Check sheet for the modelled part. Datum: model origin and axes. Units: mm. Face numbers are marked on the shaded views. A direction names the side the tool comes from. Coordinates: 2 decimals unless noted, no trailing zeros. Loops run counter-clockwise (first coordinate to the right, second up) from the corner with the lowest first, then second, coordinate; pieces in that order, holes last. Notation, with made-up numbers: (85.25, 49) -> (112.25, 49) arc R29 cw to (112.25, 77) -> close; hole circle Ø6 at (8.25, 2.25). An arc over 180 degrees is marked (long way). Use one line per item in the form item = value.
from build123d import *

# Parameters (mm, degrees)
SKETCH1_R           = 10
BOSS_EXTRUDE1_DEPTH = 10
BOSS_EXTRUDE2_DEPTH = 10
SKETCH4_R           = 2.825
CUT_EXTRUDE1_DEPTH  = 3.7
SKETCH5_R           = 1.6
CUT_EXTRUDE2_DEPTH  = 20.917820636
SKETCH7_R           = 3
CUT_EXTRUDE3_DEPTH  = 3


with BuildPart() as part:
    # Sketch1 → Boss-Extrude1 (new body)
    with BuildSketch(Plane(origin=(0, 0, 0), x_dir=(1, 0, 0), z_dir=(0, 1, 0))):
        with Locations(Location((0, 0, 0), (0, 0, 270))):
            Circle(SKETCH1_R)
    extrude(amount=BOSS_EXTRUDE1_DEPTH)

    # Sketch3 → Boss-Extrude2 (add)
    with BuildSketch(Plane(origin=(0, 10, 0), x_dir=(1, 0, 0), z_dir=(0, 1, 0))):
        with BuildLine():
            ThreePointArc((-0.292653692, 12.182759316), (-0.746983902, 11.075453202), (-0.972488982, 9.9))
            ThreePointArc((-0.972488982, 9.9), (0, 9.947649713), (0.972488982, 9.9))
            ThreePointArc((0.972488982, 9.9), (0.746983902, 11.075453202), (0.292653692, 12.182759316))
            ThreePointArc((0.292653692, 12.182759316), (0, 12.186273866), (-0.292653692, 12.182759316))
        make_face()
        with BuildLine():
            ThreePointArc((3.005067828, 11.809946574), (2.2688378, 10.866279198), (1.734561582, 9.795255532))
            ThreePointArc((1.734561582, 9.795255532), (2.683843773, 9.578763877), (3.607414487, 9.270506757))
            ThreePointArc((3.607414487, 9.270506757), (3.707405226, 10.463211508), (3.568670426, 11.652032532))
            ThreePointArc((3.568670426, 11.652032532), (3.287817341, 11.734373774), (3.005067828, 11.809946574))
        make_face()
        with BuildLine():
            ThreePointArc((6.079917215, 10.561244121), (5.116390182, 9.851202976), (4.312967649, 8.964041772))
            ThreePointArc((4.312967649, 8.964041772), (5.168639132, 8.499464945), (5.974794562, 7.953462438))
            ThreePointArc((5.974794562, 7.953462438), (6.392865264, 9.074961283), (6.580015201, 10.257127799))
            ThreePointArc((6.580015201, 10.257127799), (6.331792311, 10.41218886), (6.079917215, 10.561244121))
        make_face()
        with BuildLine():
            ThreePointArc((8.703846955, 8.529262507), (7.58448331, 8.105508096), (6.571500635, 7.468006041))
            ThreePointArc((6.571500635, 7.468006041), (7.270100171, 6.789799579), (7.899051458, 6.046546195))
            ThreePointArc((7.899051458, 6.046546195), (8.604195731, 7.013662695), (9.103350349, 8.101498821))
            ThreePointArc((9.103350349, 8.101498821), (8.906167212, 8.317779531), (8.703846955, 8.529262507))
        make_face()
        with BuildLine():
            ThreePointArc((10.682252184, 5.864704511), (9.490070008, 5.758664761), (8.342655482, 5.418102466))
            ThreePointArc((8.342655482, 5.418102466), (8.832371138, 4.576565841), (9.237471842, 3.691185281))
            ThreePointArc((9.237471842, 3.691185281), (10.177392362, 4.43219283), (10.951531647, 5.345018737))
            ThreePointArc((10.951531647, 5.345018737), (10.820012433, 5.606478546), (10.682252184, 5.864704511))
        make_face()
        with BuildLine():
            ThreePointArc((11.868403637, 2.765188211), (10.691821627, 2.984727604), (9.495073737, 2.966363017))
            ThreePointArc((9.495073737, 2.966363017), (9.739585544, 2.02390915), (9.890791199, 1.062066042))
            ThreePointArc((9.890791199, 1.062066042), (10.99577836, 1.522007499), (11.987487943, 2.192123066))
            ThreePointArc((11.987487943, 2.192123066), (11.93138683, 2.479370695), (11.868403637, 2.765188211))
        make_face()
        with BuildLine():
            ThreePointArc((12.174329886, -0.539409449), (11.100609748, -0.010573145), (9.94328581, 0.294621993))
            ThreePointArc((9.94328581, 0.294621993), (9.924459446, -0.678851624), (9.81055582, -1.645821778))
            ThreePointArc((9.81055582, -1.645821778), (10.99865778, -1.501058166), (12.134387098, -1.123352345))
            ThreePointArc((12.134387098, -1.123352345), (12.157864849, -0.831620739), (12.174329886, -0.539409449))
        make_face()
        with BuildLine():
            ThreePointArc((11.577341782, -3.804001578), (10.686116426, -3.005089732), (9.654049862, -2.398969796))
            ThreePointArc((9.654049862, -2.398969796), (9.373281592, -3.331265078), (9.002716396, -4.231646525))
            ThreePointArc((9.002716396, -4.231646525), (10.185817067, -4.412797214), (11.381334272, -4.355513852))
            ThreePointArc((11.381334272, -4.355513852), (11.48264965, -4.080934666), (11.577341782, -3.804001578))
        make_face()
        with BuildLine():
            ThreePointArc((10.1217152, -6.786468311), (9.479082735, -5.776732561), (8.6488172, -4.914640969))
            ThreePointArc((8.6488172, -4.914640969), (8.126930322, -5.736613841), (7.527186681, -6.503629408))
            ThreePointArc((7.527186681, -6.503629408), (8.6175409, -6.997259279), (9.78417995, -7.264646822))
            ThreePointArc((9.78417995, -7.264646822), (9.955818856, -7.027584338), (10.1217152, -6.786468311))
        make_face()
        with BuildLine():
            ThreePointArc((7.915407306, -9.265613737), (7.569028841, -8.119941563), (7.002141332, -7.065815706))
            ThreePointArc((7.002141332, -7.065815706), (6.277841808, -7.716504199), (5.493399966, -8.29326785))
            ThreePointArc((5.493399966, -8.29326785), (6.410141146, -9.062766634), (7.46137776, -9.63499417))
            ThreePointArc((7.46137776, -9.63499417), (7.690610523, -9.453030229), (7.915407306, -9.265613737))
        make_face()
        with BuildLine():
            ThreePointArc((5.122049862, -11.057570978), (5.097614704, -9.860931645), (4.836148674, -8.692951215))
            ThreePointArc((4.836148674, -8.692951215), (3.963154487, -9.124096741), (3.052192905, -9.467832555))
            ThreePointArc((3.052192905, -9.467832555), (3.727330549, -10.456130047), (4.585199315, -11.290758078))
            ThreePointArc((4.585199315, -11.290758078), (4.855024789, -11.177388113), (5.122049862, -11.057570978))
        make_face()
        with BuildLine():
            ThreePointArc((1.948813412, -12.029438766), (2.248133804, -10.870581538), (2.311480993, -9.6753703))
            ThreePointArc((2.311480993, -9.6753703), (1.354538128, -9.854996767), (0.384618659, -9.940211432))
            ThreePointArc((0.384618659, -9.940211432), (0.768080896, -11.074010128), (1.368957613, -12.109138111))
            ThreePointArc((1.368957613, -12.109138111), (1.659364077, -12.072770253), (1.948813412, -12.029438766))
        make_face()
        with BuildLine():
            ThreePointArc((-1.368957613, -12.109138111), (-0.768080896, -11.074010128), (-0.384618659, -9.940211432))
            ThreePointArc((-0.384618659, -9.940211432), (-1.354538128, -9.854996767), (-2.311480993, -9.6753703))
            ThreePointArc((-2.311480993, -9.6753703), (-2.248133804, -10.870581538), (-1.948813412, -12.029438766))
            ThreePointArc((-1.948813412, -12.029438766), (-1.659364077, -12.072770253), (-1.368957613, -12.109138111))
        make_face()
        with BuildLine():
            ThreePointArc((-4.585199315, -11.290758078), (-3.727330549, -10.456130047), (-3.052192905, -9.467832555))
            ThreePointArc((-3.052192905, -9.467832555), (-3.963154487, -9.124096741), (-4.836148674, -8.692951215))
            ThreePointArc((-4.836148674, -8.692951215), (-5.097614704, -9.860931645), (-5.122049862, -11.057570978))
            ThreePointArc((-5.122049862, -11.057570978), (-4.855024789, -11.177388113), (-4.585199315, -11.290758078))
        make_face()
        with BuildLine():
            ThreePointArc((-7.46137776, -9.63499417), (-6.410141146, -9.062766634), (-5.493399966, -8.29326785))
            ThreePointArc((-5.493399966, -8.29326785), (-6.277841808, -7.716504199), (-7.002141332, -7.065815706))
            ThreePointArc((-7.002141332, -7.065815706), (-7.569028841, -8.119941563), (-7.915407306, -9.265613737))
            ThreePointArc((-7.915407306, -9.265613737), (-7.690610523, -9.453030229), (-7.46137776, -9.63499417))
        make_face()
        with BuildLine():
            ThreePointArc((-9.78417995, -7.264646822), (-8.6175409, -6.997259279), (-7.527186681, -6.503629408))
            ThreePointArc((-7.527186681, -6.503629408), (-8.126930322, -5.736613841), (-8.6488172, -4.914640969))
            ThreePointArc((-8.6488172, -4.914640969), (-9.479082735, -5.776732561), (-10.1217152, -6.786468311))
            ThreePointArc((-10.1217152, -6.786468311), (-9.955818856, -7.027584338), (-9.78417995, -7.264646822))
        make_face()
        with BuildLine():
            ThreePointArc((-11.381334272, -4.355513852), (-10.185817067, -4.412797214), (-9.002716396, -4.231646525))
            ThreePointArc((-9.002716396, -4.231646525), (-9.373281592, -3.331265078), (-9.654049862, -2.398969796))
            ThreePointArc((-9.654049862, -2.398969796), (-10.686116426, -3.005089732), (-11.577341782, -3.804001578))
            ThreePointArc((-11.577341782, -3.804001578), (-11.48264965, -4.080934666), (-11.381334272, -4.355513852))
        make_face()
        with BuildLine():
            ThreePointArc((-12.134387098, -1.123352345), (-10.99865778, -1.501058166), (-9.81055582, -1.645821778))
            ThreePointArc((-9.81055582, -1.645821778), (-9.924459446, -0.678851624), (-9.94328581, 0.294621993))
            ThreePointArc((-9.94328581, 0.294621993), (-11.100609748, -0.010573145), (-12.174329886, -0.539409449))
            ThreePointArc((-12.174329886, -0.539409449), (-12.157864849, -0.831620739), (-12.134387098, -1.123352345))
        make_face()
        with BuildLine():
            ThreePointArc((-11.987487943, 2.192123066), (-10.99577836, 1.522007499), (-9.890791199, 1.062066042))
            ThreePointArc((-9.890791199, 1.062066042), (-9.739585544, 2.02390915), (-9.495073737, 2.966363017))
            ThreePointArc((-9.495073737, 2.966363017), (-10.691821627, 2.984727604), (-11.868403637, 2.765188211))
            ThreePointArc((-11.868403637, 2.765188211), (-11.93138683, 2.479370695), (-11.987487943, 2.192123066))
        make_face()
        with BuildLine():
            ThreePointArc((-10.951531647, 5.345018737), (-10.177392362, 4.43219283), (-9.237471842, 3.691185281))
            ThreePointArc((-9.237471842, 3.691185281), (-8.832371138, 4.576565841), (-8.342655482, 5.418102466))
            ThreePointArc((-8.342655482, 5.418102466), (-9.490070008, 5.758664761), (-10.682252184, 5.864704511))
            ThreePointArc((-10.682252184, 5.864704511), (-10.820012433, 5.606478546), (-10.951531647, 5.345018737))
        make_face()
        with BuildLine():
            ThreePointArc((-9.103350349, 8.101498821), (-8.604195731, 7.013662695), (-7.899051458, 6.046546195))
            ThreePointArc((-7.899051458, 6.046546195), (-7.270100171, 6.789799579), (-6.571500635, 7.468006041))
            ThreePointArc((-6.571500635, 7.468006041), (-7.58448331, 8.105508096), (-8.703846955, 8.529262507))
            ThreePointArc((-8.703846955, 8.529262507), (-8.906167212, 8.317779531), (-9.103350349, 8.101498821))
        make_face()
        with BuildLine():
            ThreePointArc((-6.580015201, 10.257127799), (-6.392865264, 9.074961283), (-5.974794562, 7.953462438))
            ThreePointArc((-5.974794562, 7.953462438), (-5.168639132, 8.499464945), (-4.312967649, 8.964041772))
            ThreePointArc((-4.312967649, 8.964041772), (-5.116390182, 9.851202976), (-6.079917215, 10.561244121))
            ThreePointArc((-6.079917215, 10.561244121), (-6.331792311, 10.41218886), (-6.580015201, 10.257127799))
        make_face()
        with BuildLine():
            ThreePointArc((-3.568670426, 11.652032532), (-3.707405226, 10.463211508), (-3.607414487, 9.270506757))
            ThreePointArc((-3.607414487, 9.270506757), (-2.683843773, 9.578763877), (-1.734561582, 9.795255532))
            ThreePointArc((-1.734561582, 9.795255532), (-2.2688378, 10.866279198), (-3.005067828, 11.809946574))
            ThreePointArc((-3.005067828, 11.809946574), (-3.287817341, 11.734373774), (-3.568670426, 11.652032532))
        make_face()
    extrude(amount=-BOSS_EXTRUDE2_DEPTH)

    # Sketch4 → Cut-Extrude1 (cut)
    with BuildSketch(Plane.XZ):
        with Locations(Location((0, 0, 0), (0, 0, 270))):
            Circle(SKETCH4_R)
    extrude(amount=-CUT_EXTRUDE1_DEPTH, mode=Mode.SUBTRACT)

    # Sketch5 → Cut-Extrude2 (cut, through all)
    with BuildSketch(Plane(origin=(0, 10, 0), x_dir=(1, 0, 0), z_dir=(0, 1, 0))):
        with Locations(Location((0, 0, 0), (0, 0, 270))):
            Circle(SKETCH5_R)
    extrude(amount=-CUT_EXTRUDE2_DEPTH, mode=Mode.SUBTRACT)

    # Sketch7 → Cut-Extrude3 (cut)
    with BuildSketch(Plane(origin=(0, 10, 0), x_dir=(1, 0, 0), z_dir=(0, 1, 0))):
        with Locations(Location((0, 0, 0), (0, 0, 270))):
            Circle(SKETCH7_R)
    extrude(amount=-CUT_EXTRUDE3_DEPTH, mode=Mode.SUBTRACT)


solid = part.part
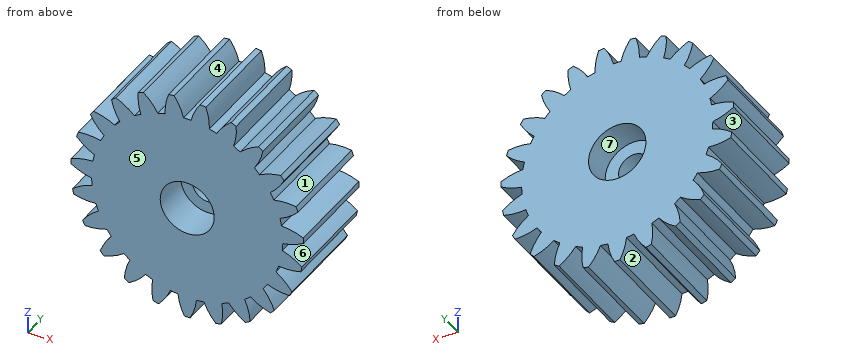
(1) Section check B-B, the plane z = 5.5. Record the boundary of the cut face in (x, y).
Established:
outline = (-9.25, 0) -> (9.25, 0) -> (9.25, 10) -> (-9.25, 10) -> close
(2) Go/stop test with flat-tipped pins: P1, Ø1.8, axis at x = 0.5, z = 0, coming from the +Y side; P2, Ø6, axis at x = -8, y = 2, coming from the -Z side; P3, Ø5, axis at x = 0, z = 0, coming from the -Y side; P4, Ø3.5, axis at x = 0, z = 0, coming from the +Y side. Record where each tip stops, or that it passes through.
Established:
P1 = through
P2 = -10.56
P3 = 3.7
P4 = 7
(3) Section check A-A, the plane x = 0. Record the boundary of the cut face in (y, z) (3 decimals).
Established:
outline = (0, -12.186) -> (10, -12.186) -> (10, -3) -> (7, -3) -> (7, -1.6) -> (3.7, -1.6) -> (3.7, -2.825) -> (0, -2.825) -> close; (0, 2.825) -> (3.7, 2.825) -> (3.7, 1.6) -> (7, 1.6) -> (7, 3) -> (10, 3) -> (10, 10) -> (0, 10) -> close
(4) Tool access check on the marked faces 1, 2, 3 and 4. Record the directions out of +Z, -Z, +X, -X, +Y, -Y that give a thin tool (end or side, any length) a straight path to the whole face; none if there is none.
Established:
face_1 = +Y, -Y
face_2 = -Z, +Y, -Y
face_3 = -X, +Y, -Y
face_4 = +Z, +Y, -Y
(5) Scan lines: line 1 along X through (y, z) = (6.75, 10.5); line 2 along X through (y, z) = (5.75, -7.75); line 3 along Z through (x, y) = (11.25, 8.75). Record each from-to range of solid material in increasing order.
Established:
line_1 = -5.14 to -3.76, -2.29 to -0.54, 0.54 to 2.29, 3.76 to 5.14
line_2 = -8.97 to -6.97, -6.32 to 6.32, 6.97 to 8.97
line_3 = -2.91 to -1.67, 0.07 to 1.44, 3.47 to 4.37
(6) Mould release check, pull along X, two halves, no side actions. Record for the marked faces 5, 6 and 7: +X half, -X half, draft (parallel to the pull), parting line (faces both ways), or undercut.
Established:
face_5 = draft
face_6 = +X half
face_7 = undercut
